Design review of the part built by this model. Coordinates are the model's own, in mm. Round coordinates to 2 decimals unless told otherwise and drop trailing zeros. Write each loop counter-clockwise with the first axis right and the second up, starting at its lowest first coordinate (ties: lowest second). Pieces come first, ordered by that corner, then holes. Notation, with made-up numbers: (11, -8.5) - (64, -8.5) arc R11 cw to (64, -2.5) - close; hole circle Ø2 at (8.5, 59.25). An arc over 180 degrees is marked (long way). Use one line per item in the form item = value.
```python
from build123d import *

# Parameters (mm, degrees)
BOSS_EXTRUDE6_DEPTH = 1.75


with BuildPart() as part:
    # Sketch2 → Boss-Extrude6 (new, symmetric)
    with BuildSketch(Plane(origin=(0, 0, 0), x_dir=(1, 0, 0), z_dir=(0, 1, 0))):
        with BuildLine():
            Line((-10.739531219, 15.234845975), (10.464592886, 15.234845975))
            ThreePointArc((10.464592886, 15.234845975), (14.498154651, 11.463496319), (17.237579405, 6.668889894))
            add(Edge.make_bspline(
                [(10.464592886, 9.300123426), (10.269158267, -0.534114199), (17.237579405, 6.668889894)],
                knots=[0, 0, 0, 1, 1, 1], degree=2))
            ThreePointArc((10.464592886, 9.300123426), (-13.973393874, 0.862707152), (9.241114219, -10.516739418))
            add(Edge.make_bspline(
                [(9.241114219, -10.516739418), (6.173157196, -1.690016533), (14.753630457, -11.391595632)],
                knots=[0, 0, 0, 1, 1, 1], degree=2))
            ThreePointArc((14.753630457, -11.391595632), (-13.463658356, -12.890615438), (-10.739531219, 15.234845975))
        make_face()
    extrude(amount=BOSS_EXTRUDE6_DEPTH, both=True)


solid = part.part
```
Q1. Draft analysis for pull direction X (two halves, no side actions). For faces 1 (the cylindrical face through (14.45, 0.024, -11.524)), 2 (the cylindrical face through (-13.15, 0.02, 13.21)), 3 (the cylindrical face through (-13.937, 0.024, -1.323)), 4 (the flat face through (-13, 1.75, 7)), state which applies: released by +X, released by -X, zero draft, split by the parting line, or undercut.
Calculated:
face_1 = released by +X
face_2 = split by the parting line
face_3 = undercut
face_4 = zero draft
Q2. We need section A-A on x = 0. Write out the cut boundary in (y, z).
Calculated:
outline = (-1.75, -15.23) - (1.75, -15.23) - (1.75, -14) - (-1.75, -14) - close; (-1.75, 14) - (1.75, 14) - (1.75, 18.64) - (-1.75, 18.64) - close
Q3. We need section C-C on z = 0. Write out the cut boundary in (x, y), then the cut area to 3 significant figures.
Calculated:
outline = (-18.64, -1.75) - (-14, -1.75) - (-14, 1.75) - (-18.64, 1.75) - close
area = 16.2 mm2
Q4. To check wall thickness, follow line 1 along Z through (x, y) = (-0.5, 1.45); line 2 along X through (y, z) = (0.4, 0); line 3 along Z through (x, y) = (6.5, -1.4). State the ranges of each line that lie inside material, in increasing order. Write a range as from..to.
Calculated:
line_1 = -15.23..-13.99, 13.99..18.63
line_2 = -18.64..-14
line_3 = -15.23..-12.4, 12.4..17.47
Q5. For P1, Ø17, axis at x = 0, z = 0, coming from the -Y side; P2, Ø1, axis at x = 13, y = 1, coming from the +Z side, all flat-tipped, find the tip position at first contact; note any pin that passes through.
Calculated:
P1 = through
P2 = 13.83
Q6. We need section D-D on x = -16. Write out the cut boundary in (y, z).
Calculated:
outline = (-1.75, -9.56) - (1.75, -9.56) - (1.75, 9.56) - (-1.75, 9.56) - close
Q7. We need section B-B on z = 12. Write out the cut boundary in (x, y).
Calculated:
outline = (-14.26, -1.75) - (-7.21, -1.75) - (-7.21, 1.75) - (-14.26, 1.75) - close; (7.21, -1.75) - (14.26, -1.75) - (14.26, 1.75) - (7.21, 1.75) - close
